Study the drawing (mm; zero at the part's minimum x, y, z) and answer. A direction names the side the tool comes from. Coordinates: 2 decimals unless noted, no trailing zeros. Order: outer loops, then holes, each group sorted by start corner. A loop starts at its lowest first (then second) coordinate and runs counter-clockwise, first axis right, second up.
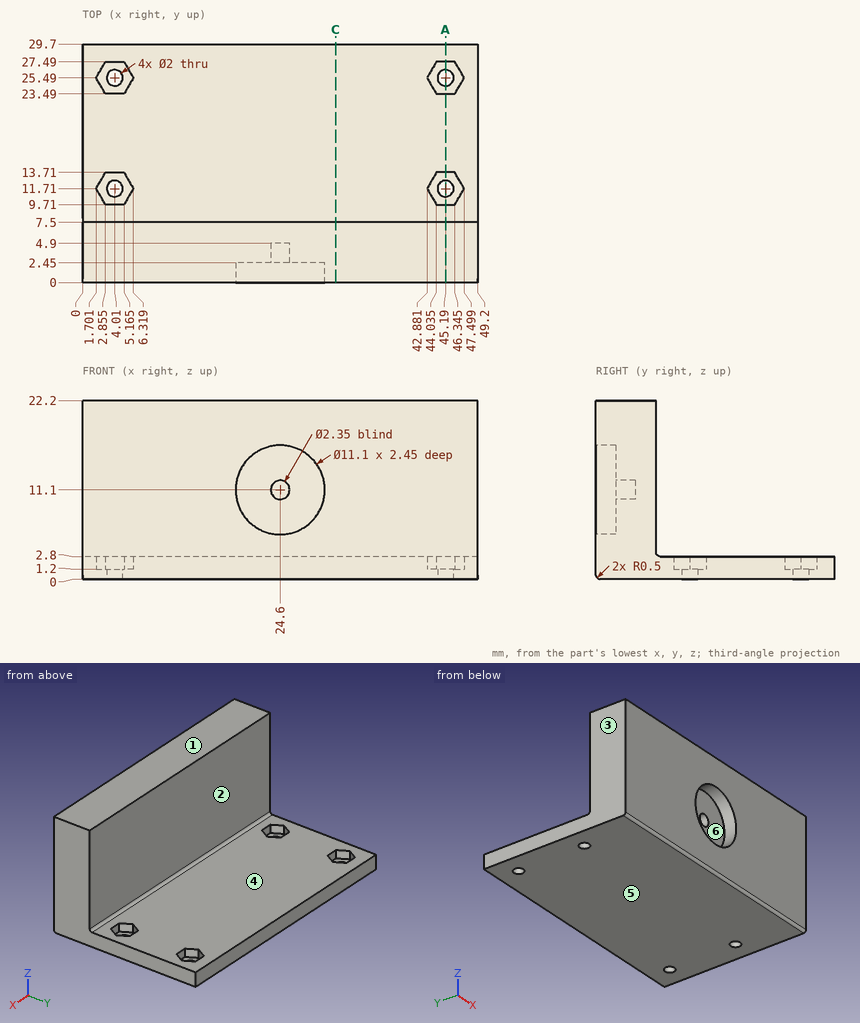
(1) Given pin 1 Ø1.2 at (x, z) = (24.5, 11) entering from -Y; pin 2 Ø1.2 at (x, y) = (45.19, 25.49) entering from +Z; pin 3 Ø2 at (x, z) = (37, 5) entering from +Y; pin 4 Ø3 at (x, y) = (44.5, 12) entering from +Z, each flat-ended and moving along its own axis, determine where each tip first touches the part or whether it passes through.
(2) Find section A-A on x = 45.19. Determine the outline of the cut face in (y, z), then the cut area to 3 significant figures.
(3) A tool of negligible diameter and unlimited length cuts with its end or side. For the marked faces 1 and 2, from which of +Z, -Z, +X, -X, +Y, -Y can it reach the whole face along a straight path? Write none if from no direction.
(4) Find the intervals of material crossed by probe 1 along Y at (x, z) = (45.19, 0.85); probe 2 along Z at (x, y) = (24.6, 1.2); probe 3 along Z at (x, y) = (8.5, 14.5), in increasing order.
(5) The mould has two halves that part along Z. Classify the marked faces 3, 4, 5 and 6: pulls with the +Z half, pulls with the -Z half, needs draft (parallel to the pull), parting line crosses it, or undercut.
(6) Find section C-C on x = 31.5. Determine the outline of the cut face in (y, z).
Resolved:
1. pin 1: stops at y = 4.9
1. pin 2: passes through
1. pin 3: stops at y = 7.5
1. pin 4: stops at z = 2.8
2. outline: (0, 0.5) arc R0.5 ccw to (0.5, 0) - (10.71, 0) - (10.71, 1.2) - (9.71, 1.2) - (9.71, 2.8) - (8, 2.8) arc R0.5 cw to (7.5, 3.3) - (7.5, 22.2) - (0, 22.2) - close; (12.71, 0) - (24.49, 0) - (24.49, 1.2) - (23.49, 1.2) - (23.49, 2.8) - (13.71, 2.8) - (13.71, 1.2) - (12.71, 1.2) - close; (26.49, 0) - (29.7, 0) - (29.7, 2.8) - (27.49, 2.8) - (27.49, 1.2) - (26.49, 1.2) - close
2. area: 211 mm2
3. face 1: +Z, +X, -X, +Y, -Y
3. face 2: +Z, +X, -X, +Y
4. probe 1: y = 0 to 10.71, 12.71 to 24.49, 26.49 to 29.7
4. probe 2: z = 0 to 5.55, 16.65 to 22.2
4. probe 3: z = 0 to 2.8
5. face 3: needs draft
5. face 4: pulls with the +Z half
5. face 5: pulls with the -Z half
5. face 6: undercut
6. outline: (0, 0.5) arc R0.5 ccw to (0.5, 0) - (29.7, 0) - (29.7, 2.8) - (8, 2.8) arc R0.5 cw to (7.5, 3.3) - (7.5, 22.2) - (0, 22.2) - close
